The model under review builds one solid part; all positions refer to its coordinate system, in mm. A direction names the side the tool comes from. Round coordinates to 2 decimals unless told otherwise and drop trailing zeros. Write each loop counter-clockwise with the first axis right and the second up, starting at its lowest first coordinate (ties: lowest second). Pieces come first, ordered by that corner, then holes. Notation, with made-up numbers: M 72,13.25 L 92,13.25 A11 ccw 92,22.25 Z; hole C 72.25,47.25 d7. An arc over 180 degrees is marked long. One line per item, written item: value. Start each with the question number.
1) Wall thickness on probe 1 along X at (y, z) = (2.9, -23.5); probe 2 along Y at (x, z) = (-83.5, -14); probe 3 along Z at (x, y) = (-23, 3.4): over which ranges is each line inside the solid? List them lowest first.
2) Take a section at A-A, the plane z = -25. Write out the cut boundary in (x, y).
3) Take a section at B-B, the plane y = 2.9. Write out the cut boundary in (x, z).
4) Tool access review of faces 1 (the face through (-23.464, 3, -24)), 2 (the face through (-59, 0, -13)), 3 (the face through (-46, 3, -21.809)): name each direction out of +Z, -Z, +X, -X, +Y, -Y from which nothing blocks a thin tool from reaching the whole face with its end or side.
5) For P1, Ø0.6, axis at x = -95, y = 3, coming from the +Z side; P2, Ø1.6, axis at x = -69, y = 2.5, coming from the +Z side; P3, Ø1.5, axis at x = -57.5, y = 3, coming from the -Z side, all flat-tipped, find the tip position at first contact; note any pin that passes through.
6) Mouldability with a two-part tool opening along X and no side actions: class faces 4 (the face through (-21, 3, -21.809)), 5 (the face through (-18.464, 1, -12)), 6 (the face through (-59, 2, -13)) as +X half, -X half, draft (parallel to the pull), parting line (faces both ways), or undercut.
7) Take a section at C-C, the plane x = -69.5. Write out the cut boundary in (y, z).
8) Take a section at D-D, the plane z = -13.75. Write out the cut boundary in (x, y).
from build123d import *

# Parameters (mm, degrees)
SKETCH_1_W      = 79
SKETCH_1_H      = 29
EXTRUDE_1_DEPTH = 2
SKETCH_2_W      = 5
SKETCH_2_H      = 5
EXTRUDE_3_DEPTH = 4
SKETCH_3_W      = 5
SKETCH_3_H      = 5
EXTRUDE_4_DEPTH = 4


with BuildPart() as part:
    # 草图1 → 凸台-拉伸1 (new body)
    with BuildSketch(Plane(origin=(0, 0, 0), x_dir=(1, 0, 0), z_dir=(0, 1, 0))):
        with Locations((-57.963659684, 12.309109642)):
            Rectangle(SKETCH_1_W, SKETCH_1_H)
    extrude(amount=EXTRUDE_1_DEPTH)

    # 草图2 → 凸台-拉伸3 (add)
    with BuildSketch(Plane(origin=(0, 0, 0), x_dir=(1, 0, 0), z_dir=(0, 1, 0))):
        with Locations((-94.963659684, 24.309109642)):
            Rectangle(SKETCH_2_W, SKETCH_2_H)
        with Locations((-20.963659684, 24.309109642)):
            Rectangle(SKETCH_2_W, SKETCH_2_H)
    extrude(amount=EXTRUDE_3_DEPTH)

    # 草图3 → 凸台-拉伸4 (add)
    with BuildSketch(Plane(origin=(0, 0, 0), x_dir=(1, 0, 0), z_dir=(0, 1, 0))):
        with Locations((-69.963659684, 24.309109642)):
            Rectangle(SKETCH_3_W, SKETCH_3_H)
        with Locations((-46.003915764, 24.309109642)):
            Rectangle(SKETCH_3_W, SKETCH_3_H)
    extrude(amount=EXTRUDE_4_DEPTH)


solid = part.part
Checked values:
1. probe 1: x = -97.46 to -92.46, -72.46 to -67.46, -48.5 to -43.5, -23.46 to -18.46
1. probe 2: y = 0 to 2
1. probe 3: z = -26.81 to -21.81
2. outline: M -97.46,0 L -18.46,0 L -18.46,4 L -23.46,4 L -23.46,2 L -43.5,2 L -43.5,4 L -48.5,4 L -48.5,2 L -67.46,2 L -67.46,4 L -72.46,4 L -72.46,2 L -92.46,2 L -92.46,4 L -97.46,4 Z
3. outline: M -97.46,-26.81 L -92.46,-26.81 L -92.46,-21.81 L -97.46,-21.81 Z; M -72.46,-26.81 L -67.46,-26.81 L -67.46,-21.81 L -72.46,-21.81 Z; M -48.5,-26.81 L -43.5,-26.81 L -43.5,-21.81 L -48.5,-21.81 Z; M -23.46,-26.81 L -18.46,-26.81 L -18.46,-21.81 L -23.46,-21.81 Z
4. face 1: +Z, -Z, +Y
4. face 2: +Z, -Z, +X, -X, -Y
4. face 3: +Z, +X, -X, +Y
5. P1: stops at z = -21.81
5. P2: stops at z = 2.19
5. P3: passes through
6. face 4: draft
6. face 5: +X half
6. face 6: undercut
7. outline: M 0,-26.81 L 4,-26.81 L 4,-21.81 L 2,-21.81 L 2,2.19 L 0,2.19 Z
8. outline: M -97.46,0 L -18.46,0 L -18.46,2 L -97.46,2 Z
